from build123d import *

# Parameters (mm, degrees)
BASPROSKE_W         = 8
BASPROSKE_H         = 20.25
TOOTHCUT_DEPTH      = 30.734239523
TEETHCUTS_COUNT     = 25
TEETHCUTS_ANGLE     = 345.6
BORSKE_R            = 0.5
BORE_DEPTH          = 50.0000508
SKETCH_1_R          = 10.5
CUT_EXTRUDE_1_DEPTH = 2.2
SKETCH_2_R          = 4.4
SKETCH_2_R_2        = 1.05
CUT_EXTRUDE_2_DEPTH = 30.207030593


with BuildPart() as part:
    # BasProSke → Base-Revolve (revolve)
    with BuildSketch(Plane(origin=(0, 0, 0), x_dir=(1, 0, 0), z_dir=(0, 1, 0)), mode=Mode.PRIVATE) as base_revolve_sk:
        with Locations((4, 10.125)):
            Rectangle(BASPROSKE_W, BASPROSKE_H)
    revolve(base_revolve_sk.sketch.rotate(Axis((-10, 0, 0), (1, 0, 0)), 180), axis=Axis((-10, 0, 0), (1, 0, 0)))

    # TooCutSke → ToothCut (cut, through all)
    with BuildSketch(Plane(origin=(0, 0, 0), x_dir=(0, 0, -1), z_dir=(1, 0, 0))):
        with BuildLine():
            ThreePointArc((0.713909619, 16.858891098), (0, 16.874), (-0.713909619, 16.858891098))
            ThreePointArc((-0.713909619, 16.858891098), (-1.221902209, 18.597177626), (-2.131751691, 20.163022588))
            ThreePointArc((-2.131751691, 20.163022588), (0, 20.2754), (2.131751691, 20.163022588))
            ThreePointArc((2.131751691, 20.163022588), (1.221902209, 18.597177626), (0.713909619, 16.858891098))
        make_face()
    toothcut = extrude(amount=TOOTHCUT_DEPTH, mode=Mode.SUBTRACT)

    # TeethCuts: ToothCut ×25 about axis
    teethcuts_axis = Axis((-10, 0, 0), (1, 0, 0))
    for i in range(1, TEETHCUTS_COUNT):
        add(toothcut.rotate(teethcuts_axis, i * TEETHCUTS_ANGLE / (TEETHCUTS_COUNT - 1)), mode=Mode.SUBTRACT)

    # BorSke → Bore (cut, symmetric)
    with BuildSketch(Plane(origin=(0, 0, 0), x_dir=(0, 0, -1), z_dir=(1, 0, 0))):
        with Locations(Location((0, 0, 0), (0, 0, 180))):
            Circle(BORSKE_R)
    extrude(amount=BORE_DEPTH, both=True, mode=Mode.SUBTRACT)

    # Sketch 1 → Cut-Extrude 1 (cut)
    with BuildSketch(Plane(origin=(8, 0, 0), x_dir=(0, 0, -1), z_dir=(1, 0, 0))):
        Circle(SKETCH_1_R)
    extrude(amount=-CUT_EXTRUDE_1_DEPTH, mode=Mode.SUBTRACT)

    # Sketch 2 → Cut-Extrude 2 (cut, through all)
    with BuildSketch(Plane(origin=(5.8, 0, 0), x_dir=(0, 0, -1), z_dir=(1, 0, 0))):
        Circle(SKETCH_2_R)
        with Locations((0, 7.1)):
            Circle(SKETCH_2_R_2)
        with Locations((7.1, 0)):
            Circle(SKETCH_2_R_2)
        with Locations((0, -7.1)):
            Circle(SKETCH_2_R_2)
        with Locations((-7.1, 0)):
            Circle(SKETCH_2_R_2)
    extrude(amount=-CUT_EXTRUDE_2_DEPTH, mode=Mode.SUBTRACT)


solid = part.part
Could you check a few things on this model? Use its own coordinates, in mm. A direction names the side the tool comes from. Give positions to 0.01 mm unless a question says otherwise; leave off trailing zeros.
Item 1: If we mould it in two halves opening along Z, with no side actions, what happens to faces 4 (the face through (3.94, -17.75, -5.71)), 5 (the face through (5.8, 0, -5)), 6 (the face through (3.94, -12.76, 13.53)), 7 (the face through (3.9, 6.9, -17.3))? For each: pulls with the +Z half, pulls with the -Z half, needs draft (parallel to the pull), parting line crosses it, or undercut.
Item 2: For faces 1 (the face through (3.94, -16.81, -7.95)), 2 (the face through (3.94, 12.29, -11.56)), 3 (the face through (3.94, -9.03, -16.31)), which set-ups out of +Z, -Z, +X, -X, +Y, -Y let a thin tool reach every point of the face, with its end or its side?
Item 3: I need wall thicknesses on line 1 (Y direction, x = 2.2, z = 0); line 2 (Y direction, x = 7.2, z = 0); line 3 (Z direction, x = 3.5, y = 15). Which ranges of each line are inside material? Lowest first, please.
Item 4: I'm going to push flat-ended pins straight in: pin 1 (1.9 mm diameter, centred on y = 0, z = 7.1, fed in from -X); pin 2 (12 mm diameter, centred on y = -3.5, z = 5.5, fed in from -X); pin 3 (2 mm diameter, centred on x = 6, z = -8, fed in from +Y); pin 4 (3 mm diameter, centred on x = 1, y = 6.5, fed in from -Z). Where does each tip first touch, or does it pass through?
Item 5: If we section it at A-A, the plane x = 5: Count the separate pieces of the cut face and the enclosed holes in it, plus the area to 4 significant figures.
Values:
1. face 4: undercut
1. face 5: undercut
1. face 6: pulls with the +Z half
1. face 7: pulls with the -Z half
2. face 1: +X, -X, -Y
2. face 2: +X, -X
2. face 3: -Z, +X, -X
3. line 1: y = -20.25 to -8.15, -6.05 to -4.4, 4.4 to 6.05, 8.15 to 16.87
3. line 2: y = -20.25 to -10.5, 10.5 to 16.87
3. line 3: z = -12.03 to -9.24, -7.73 to 7.73, 9.24 to 12.03
4. pin 1: passes through
4. pin 2: stops at x = 0
4. pin 3: stops at y = 18.98
4. pin 4: stops at z = -18.33
5. separate pieces: 1
5. enclosed holes: 5
5. area: 1,000 mm2
